Geometry: see drawing. Coordinates: mm, zero at the bounding-box minimum. A direction names the side the tool comes from. Coordinates: 2 decimals unless noted, no trailing zeros. Order: outer loops, then holes, each group sorted by start corner. A loop starts at its lowest first (then second) coordinate and runs counter-clockwise, first axis right, second up.
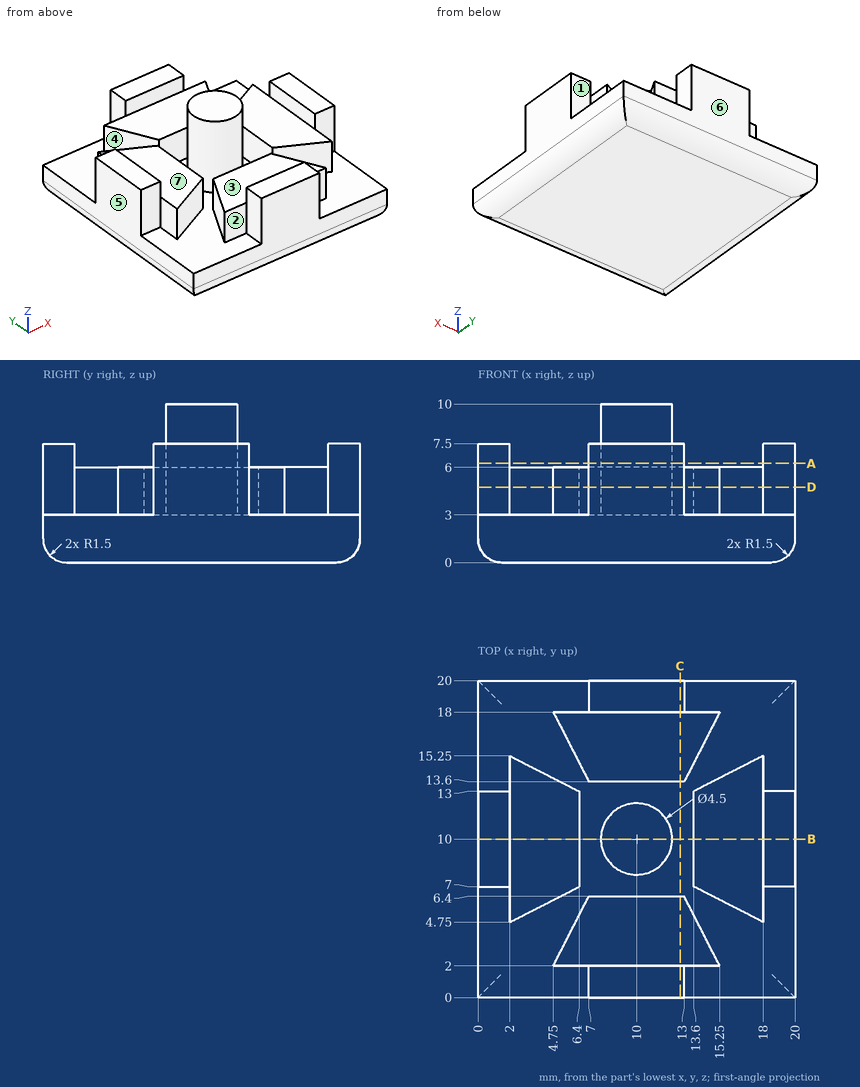
Q1. Section query D-D on z = 4.75. Give the number of separate pieces and of enclosed holes in the cut face, plus the area to 3 significant figures.
Solutions:
separate pieces: 5
enclosed holes: 0
area: 209 mm2
Q2. Section query C-C on x = 12.75. Output: boundary loops of the cut face in (y, z), plus the area to 3 significant figures.
Solutions:
outline: (0, 1.5) arc R1.5 ccw to (1.5, 0) - (18.5, 0) arc R1.5 ccw to (20, 1.5) - (20, 7.5) - (18, 7.5) - (18, 6) - (13.6, 6) - (13.6, 3) - (6.4, 3) - (6.4, 6) - (2, 6) - (2, 7.5) - (0, 7.5) - close
area: 103 mm2
Q3. Material intervals for line 1 along X through (y, z) = (7.5, 5); line 2 along Y through (x, z) = (8.75, 7); line 3 along Z through (x, y) = (18, 2.25), sorted ascending.
Solutions:
line 1: x = 0 to 6.4, 13.6 to 20
line 2: y = 0 to 2, 8.13 to 11.87, 18 to 20
line 3: z = 0 to 3
Q4. Section query A-A on z = 6.25. Output: boundary loops of the cut face in (x, y), plus the area to 3 significant figures.
Solutions:
outline: (0, 7) - (2, 7) - (2, 13) - (0, 13) - close; (7, 0) - (13, 0) - (13, 2) - (7, 2) - close; (7, 18) - (13, 18) - (13, 20) - (7, 20) - close; circle Ø4.5 at (10, 10); (18, 7) - (20, 7) - (20, 13) - (18, 13) - close
area: 63.9 mm2
Q5. Pull-direction query (X, two-part tool) for the marked faces 5, 6 and 7; classes: pulls with the +X half, pulls with the -X half, needs draft (parallel to the pull), parting line crosses it, or undercut.
Solutions:
face 5: pulls with the -X half
face 6: needs draft
face 7: undercut
Q6. Section query B-B on y = 10. Output: boundary loops of the cut face in (x, z), plus the area to 3 significant figures.
Solutions:
outline: (0, 1.5) arc R1.5 ccw to (1.5, 0) - (18.5, 0) arc R1.5 ccw to (20, 1.5) - (20, 7.5) - (18, 7.5) - (18, 6) - (13.6, 6) - (13.6, 3) - (12.25, 3) - (12.25, 10) - (7.75, 10) - (7.75, 3) - (6.4, 3) - (6.4, 6) - (2, 6) - (2, 7.5) - (0, 7.5) - close
area: 135 mm2
Q7. Set-up query: the marked faces 1, 2, 3 and 4. Return all of +Z, -Z, +X, -X, +Y, -Y with unobstructed straight access to the full face (end or side cutting, diameter ignored); none if empty.
Solutions:
face 1: +Z, +X, +Y
face 2: +Z, -X, -Y
face 3: +Z, +X, -X
face 4: +Z
Q8. Pin query (flat end, axial travel): P1, Ø0.7, axis at y = 5.5, z = 4.5, coming from the +X side; P2, Ø1, axis at x = 9, y = 15, coming from the +Z side; P3, Ø0.6, axis at x = 19, z = 6.5, coming from the +Y side. Return the tip coordinate at first contact, or that it passes through.
Solutions:
P1: stops at x = 18
P2: stops at z = 6
P3: stops at y = 13
